Autodesk Fusion 360 part; units mm, degrees
sketch "Sketch2" plane through (0, 0, 0) normal (0, 1, 0) x (1, 0, 0)
  line L0 (-8.5, -11.5) -> (8.5, -11.5)
  line L1 (11.5, -8.5) -> (11.5, 8.5)
  line L2 (8.5, 11.5) -> (-8.5, 11.5)
  line L3 (-11.5, 8.5) -> (-11.5, -8.5)
  line L4 (-11.5, -11.5) -> (11.5, 11.5) construction
  line L5 (11.5, -11.5) -> (-11.5, 11.5) construction
  line L6 (-8.5, 8.5) -> (8.5, 8.5) construction
  line L7 (8.5, 8.5) -> (8.5, -8.5) construction
  line L8 (8.5, -8.5) -> (-8.5, -8.5) construction
  line L9 (-8.5, -8.5) -> (-8.5, 8.5) construction
  line L10 (-8.5, 8.5) -> (8.5, -8.5) construction
  line L11 (8.5, 8.5) -> (-8.5, -8.5) construction
  circle A0 centre (-8.5, 8.5) radius 1.5
  circle A1 centre (8.5, 8.5) radius 1.5
  circle A2 centre (8.5, -8.5) radius 1.5
  circle A3 centre (-8.5, -8.5) radius 1.5
  arc A4 (-8.5, 11.5) -> (-11.5, 8.5) centre (-8.5, 8.5) ccw
  arc A5 (11.5, 8.5) -> (8.5, 11.5) centre (8.5, 8.5) ccw
  arc A6 (8.5, -11.5) -> (11.5, -8.5) centre (8.5, -8.5) ccw
  arc A7 (-11.5, -8.5) -> (-8.5, -11.5) centre (-8.5, -8.5) ccw
  line L12 (-2.5, -2.1) -> (2.5, -2.1)
  line L13 (2.5, -2.1) -> (2.5, 2.1)
  line L14 (2.5, 2.1) -> (-2.5, 2.1)
  line L15 (-2.5, 2.1) -> (-2.5, -2.1)
  line L16 (-2.5, -2.1) -> (2.5, 2.1) construction
  line L17 (2.5, -2.1) -> (-2.5, 2.1) construction
  circle A8 centre (-4.12, 6.5) radius 0.5
  circle A9 centre (-1.58, 6.5) radius 0.5
  circle A10 centre (0.96, 6.5) radius 0.5
  circle A11 centre (3.5, 6.5) radius 0.5
  line L18 (-4.12, 6.5) -> (-1.58, 6.5) construction
  line L19 (-1.58, 6.5) -> (0.96, 6.5) construction
  line L20 (0.96, 6.5) -> (3.5, 6.5) construction
  circle A12 centre (2.14, -6.5) radius 0.5
  circle A13 centre (-0.4, -6.5) radius 0.5
  circle A14 centre (-2.94, -6.5) radius 0.5
  line L21 (-2.94, -6.5) -> (-0.4, -6.5) construction
  line L22 (-0.4, -6.5) -> (2.14, -6.5) construction
  line L23 (-6.9, 3.63) -> (-5.02, 3.63)
  line L24 (-5.02, 3.63) -> (-5.02, 2.63)
  line L25 (-5.02, 2.63) -> (-6.9, 2.63)
  line L26 (-6.9, 2.63) -> (-6.9, 3.63)
  line L27 (-6.9, 0.63) -> (-5.02, 0.63)
  line L28 (-5.02, 0.63) -> (-5.02, -0.37)
  line L29 (-5.02, -0.37) -> (-6.9, -0.37)
  line L30 (-6.9, -0.37) -> (-6.9, 0.63)
  line L31 (-6.9, -2.37) -> (-5.02, -2.37)
  line L32 (-5.02, -2.37) -> (-5.02, -3.37)
  line L33 (-5.02, -3.37) -> (-6.9, -3.37)
  line L34 (-6.9, -3.37) -> (-6.9, -2.37)
  line L35 (-6.9, 2.63) -> (-6.9, 0.63) construction
  line L36 (-6.9, -0.37) -> (-6.9, -2.37) construction
  line L37 (6.22, 4.5) -> (8.1, 4.5)
  line L38 (8.1, 4.5) -> (8.1, 3.5)
  line L39 (8.1, 3.5) -> (6.22, 3.5)
  line L40 (6.22, 3.5) -> (6.22, 4.5)
  line L41 (6.22, 1) -> (8.1, 1)
  line L42 (8.1, 1) -> (8.1, 0)
  line L43 (8.1, 0) -> (6.22, 0)
  line L44 (6.22, 0) -> (6.22, 1)
  line L45 (6.22, -2.5) -> (8.1, -2.5)
  line L46 (8.1, -2.5) -> (8.1, -3.5)
  line L47 (8.1, -3.5) -> (6.22, -3.5)
  line L48 (6.22, -3.5) -> (6.22, -2.5)
  line L49 (8.1, -2.5) -> (8.1, 0) construction
  line L50 (8.1, 3.5) -> (8.1, 1) construction
  dimension "d6" = 23
  dimension "d7" = 23
  dimension "d8" = 17
  dimension "d9" = 17
  dimension "d10" = 3
  dimension "d11" = 3
  dimension "d12" = 3
  dimension "d13" = 3
  dimension "d14" = 3
  dimension "d15" = 5
  dimension "d16" = 4.2
  dimension "d21" = 1
  dimension "d25" = 2.54
  dimension "d26" = 2.54
  dimension "d27" = 2.54
  dimension "d28" = 5
  dimension "d29" = 8
  dimension "d30" = 2.54
  dimension "d31" = 2.54
  dimension "d32" = 5
  dimension "d33" = 8.56
  dimension "d34" = 1.88
  dimension "d35" = 1
  dimension "d36" = 2
  dimension "d37" = 2
  dimension "d38" = 4.6
  dimension "d39" = 8.13
  dimension "d41" = 3.4
  dimension "d42" = 2.5
  dimension "d43" = 2.5
  dimension "d44" = 8
extrude "Extrude1" add sketch "Sketch2" against normal blind 1.7 contours L0 L1 L2 L3 A4 A5 A6 A7 | L12 L13 L14 L15 | L23 L24 L25 L26 | L27 L28 L29 L30 | L31 L32 L33 L34 | L37 L38 L39 L40 | L41 L42 L43 L44 | L45 L46 L47 L48
extrude "Extrude2" add sketch "Sketch2" along normal blind 1.8 contours L12 L13 L14 L15
extrude "Extrude3" add sketch "Sketch2" along normal blind 0.8 contours L23 L24 L25 L26 | L37 L38 L39 L40 | L41 L42 L43 L44 | L45 L46 L47 L48
extrude "Extrude4" add sketch "Sketch2" along normal blind 1.22 contours L27 L28 L29 L30 | L31 L32 L33 L34
Verification items for the finished model (mm, model axes). A direction names the side the tool comes from. Give positions to 0.01 mm unless a question says otherwise; leave off trailing zeros. Write each loop counter-clockwise with the first axis right and the second up, starting at its lowest first coordinate (ties: lowest second). Pieces come first, ordered by that corner, then holes. Notation, with made-up numbers: M 31,4.25 L 53,4.25 A25 cw 53,43.25 Z; hole C -36.5,74 d8. An arc over 180 degrees is marked long. Write item = value, one per line.
(1) Sectioned sample at D-D (x = -9). Record the cut outline in (y, z).
Found:
outline = M -1.7,-11.46 L 0,-11.46 L 0,-9.91 L -1.7,-9.91 Z; M -1.7,-7.09 L 0,-7.09 L 0,7.09 L -1.7,7.09 Z; M -1.7,9.91 L 0,9.91 L 0,11.46 L -1.7,11.46 Z
(2) Material ranges on line 1 (X direction, y = -1.2, z = -8.5); line 2 (X direction, y = -0.25, z = -6.5), recorded low to high.
Found:
line_1 = -11.5 to -10, -7 to 7, 10 to 11.5
line_2 = -11.5 to -4.62, -3.62 to -2.08, -1.08 to 0.46, 1.46 to 3, 4 to 11.5
(3) Sectioned sample at A-A (x = -2.94). Record the cut outline in (y, z).
Found:
outline = M -1.7,-11.5 L 0,-11.5 L 0,6 L -1.7,6 Z; M -1.7,7 L 0,7 L 0,11.5 L -1.7,11.5 Z
(4) Sectioned sample at B-B (y = 0.45). Record the cut outline in (x, z), then the cut area to 3 significant figures.
Found:
outline = M -6.9,-3.63 L -5.02,-3.63 L -5.02,-2.63 L -6.9,-2.63 Z; M -6.9,-0.63 L -5.02,-0.63 L -5.02,0.37 L -6.9,0.37 Z; M -6.9,2.37 L -5.02,2.37 L -5.02,3.37 L -6.9,3.37 Z; M -2.5,-2.1 L 2.5,-2.1 L 2.5,2.1 L -2.5,2.1 Z; M 6.22,-4.5 L 8.1,-4.5 L 8.1,-3.5 L 6.22,-3.5 Z; M 6.22,-1 L 8.1,-1 L 8.1,0 L 6.22,0 Z; M 6.22,2.5 L 8.1,2.5 L 8.1,3.5 L 6.22,3.5 Z
area = 32.3 mm2
(5) Go/stop test with flat-tipped pins: pin 1 Ø0.6 at (x, y) = (-6, 0.5) entering from -Z; pin 2 Ø0.5 at (y, z) = (0.5, 0) entering from +X; pin 3 Ø0.5 at (x, z) = (-5.5, 0) entering from +Y. Record where each tip stops, or that it passes through.
Found:
pin_1 = -3.63
pin_2 = 8.1
pin_3 = 1.22
(6) Access from +Z, -Z, +X, -X, +Y, -Y to the whole of each face (thin tool, end or side, straight path). Record for faces 1 (the face through (-6, 1, -0.63)), 2 (the face through (-6, 1, 3.37)), 3 (the face through (-6.9, 1, 3)), 4 (the face through (0, 1, 2.1)).
Found:
face_1 = -X, +Y
face_2 = +Z, -X, +Y
face_3 = +Z, -Z, -X, +Y
face_4 = +Z, +X, -X, +Y
(7) Draft check along Z on faces 5 (the face through (-6.9, 1, 0)), 6 (the face through (1, -1, -6)), 7 (the face through (3.392, -0.838, -6.012)), 8 (the face through (10.64, -0.84, -10.6)). Enter one of: released by +Z, released by -Z, zero draft, split by the parting line, or undercut.
Found:
face_5 = zero draft
face_6 = undercut
face_7 = undercut
face_8 = released by -Z
(8) Sectioned sample at C-C (z = -1.5). Record the cut outline in (x, y).
Found:
outline = M -11.5,-1.7 L 11.5,-1.7 L 11.5,0 L 2.5,0 L 2.5,1.8 L -2.5,1.8 L -2.5,0 L -11.5,0 Z
